Read the model definition and answer for the solid it produces. Units are mm, in the model's axes. A direction names the side the tool comes from. Coordinates: 2 decimals unless noted, no trailing zeros. Loops run counter-clockwise (first coordinate to the right, second up) from the corner with the lowest first, then second, coordinate; pieces in that order, holes last. Notation, with made-up numbers: (1.25, -31.75) -> (23.25, -31.75) arc R19 cw to (23.25, -6.75) -> close; hole circle Ø10 at (88.5, 68.25). An arc over 180 degrees is marked (long way). Answer as a JSON object with one key per item and string values. Group by question number.
Q1. Each of these flat-tipped pins is pushed along its axis until it touches: P1, Ø2.5, axis at x = 3.5, z = -3, coming from the +Y side; P2, Ø1.4, axis at x = 2.5, y = -0.5, coming from the -Z side; P3, Ø2.5, axis at x = 1.5, z = 13.5, coming from the +Y side. Where does it stop, or does it pass through?
Q2. The part is cut by section A-A on z = 55.05. Write down the section's boundary in (x, y), and give its area (3 significant figures).
Q3. Straight lines are drawn through the part: line 1 along Y through (x, z) = (3.9, 24.95); line 2 along Y through (x, z) = (4.1, 7.5); line 3 along Z through (x, y) = (3.2, 12). For each, find the intervals that lie inside material, in ascending order. Write a range as [from, to].
Q4. The part is cut by section C-C on x = 1.05. Write down the section's boundary in (y, z), and give its area (3 significant figures).
Q5. For faces 4 (the flat face through (2, 1, 59)), 5 (the flat face through (2, -11.156, -3)), 6 (the cylindrical face through (2.46, -4.18, 56.45)), 7 (the flat face through (2, 0, 10)), 8 (the flat face through (2, -15, 0)), determine the directions among +Z, -Z, +X, -X, +Y, -Y from which every point of the face is accessible in a straight line to the end or side of a thin tool.
Q6. Determine the mould class of faces 1 (the cylindrical face through (2.46, 14.82, 56.45)), 2 (the flat face through (2, -1.752, -3)), 3 (the flat face through (0, -3, 35)) for opening direction Y: released by +Y, released by -Y, zero draft, split by the parting line, or undercut.
Q7. The part is cut by section D-D on z = 9.5. Write down the section's boundary in (x, y).
Q8. The part is cut by section B-B on y = -3.5. Write down the section's boundary in (x, z), and give its area (3 significant figures).
from build123d import *

# Parameters (mm, degrees)
SKETCH1_R           = 1.4
BOSS_EXTRUDE1_DEPTH = 5


with BuildPart() as part:
    # Sketch1 → Boss-Extrude1 (new body)
    with BuildSketch(Plane(origin=(0, 0, 0), x_dir=(0, 0, -1), z_dir=(1, 0, 0))):
        Polygon((0, 0), (-21, 0), (-21, 18.45912049), (-59, 18.45912049), (-59, 3.45912049), (-59, -16.54087951), (0, -16.54087951), (0, -13.963518408), (5, -13.963518408), (5, -11.15648618), (0, -11.15648618), (0, -8.024983971), (5, -8.024983971), (5, -1.752077979), (0, -1.752077979), align=None)
        with Locations((-24.95, -4.24087951)):
            Circle(SKETCH1_R, mode=Mode.SUBTRACT)
        with Locations((-55.05, -4.24087951)):
            Circle(SKETCH1_R, mode=Mode.SUBTRACT)
        with Locations((-24.95, 14.75912049)):
            Circle(SKETCH1_R, mode=Mode.SUBTRACT)
        with Locations((-55.05, 14.75912049)):
            Circle(SKETCH1_R, mode=Mode.SUBTRACT)
    extrude(amount=BOSS_EXTRUDE1_DEPTH)


solid = part.part
Final values:
{
 "1": {"P1": "stops at y = -1.75", "P2": "stops at z = 0", "P3": "stops at y = 0"},
 "2": {"outline": "(0, -16.54) -> (5, -16.54) -> (5, -5.64) -> (0, -5.64) -> close; (0, -2.84) -> (5, -2.84) -> (5, 13.36) -> (0, 13.36) -> close; (0, 16.16) -> (5, 16.16) -> (5, 18.46) -> (0, 18.46) -> close", "area": "147 mm2"},
 "3": {"line 1": "y = [-16.54, -5.64], [-2.84, 13.36], [16.16, 18.46]", "line 2": "y = [-16.54, 0]", "line 3": "z = [21, 59]"},
 "4": {"outline": "(-16.54, 0) -> (-13.96, 0) -> (-13.96, -5) -> (-11.16, -5) -> (-11.16, 0) -> (-8.02, 0) -> (-8.02, -5) -> (-1.75, -5) -> (-1.75, 0) -> (0, 0) -> (0, 21) -> (18.46, 21) -> (18.46, 59) -> (-16.54, 59) -> close; hole circle Ø2.8 at (-4.24, 24.95); hole circle Ø2.8 at (-4.24, 55.05); hole circle Ø2.8 at (14.76, 24.95); hole circle Ø2.8 at (14.76, 55.05)", "area": "1,700 mm2"},
 "5": {"face 4": "+Z, +X, -X, +Y, -Y", "face 5": "-Z, +X, -X", "face 6": "+X, -X", "face 7": "-Z, +X, -X, +Y", "face 8": "-Z, +X, -X, -Y"},
 "6": {"face 1": "undercut", "face 2": "released by +Y", "face 3": "zero draft"},
 "7": {"outline": "(0, -16.54) -> (5, -16.54) -> (5, 0) -> (0, 0) -> close"},
 "8": {"outline": "(0, -5) -> (5, -5) -> (5, 23.76) -> (0, 23.76) -> close; (0, 26.14) -> (5, 26.14) -> (5, 53.86) -> (0, 53.86) -> close; (0, 56.24) -> (5, 56.24) -> (5, 59) -> (0, 59) -> close", "area": "296 mm2"}
}
